Input: dimensioned drawing with shaded views. Units: mm. Origin: part minimum x, y, z. A direction names the side the tool comes from. Give positions to 0.01 mm unless a question says otherwise; leave off trailing zeros. Loops run counter-clockwise (first coordinate to the right, second up) from the corner with the lowest first, then second, coordinate; pieces in that order, holes last.
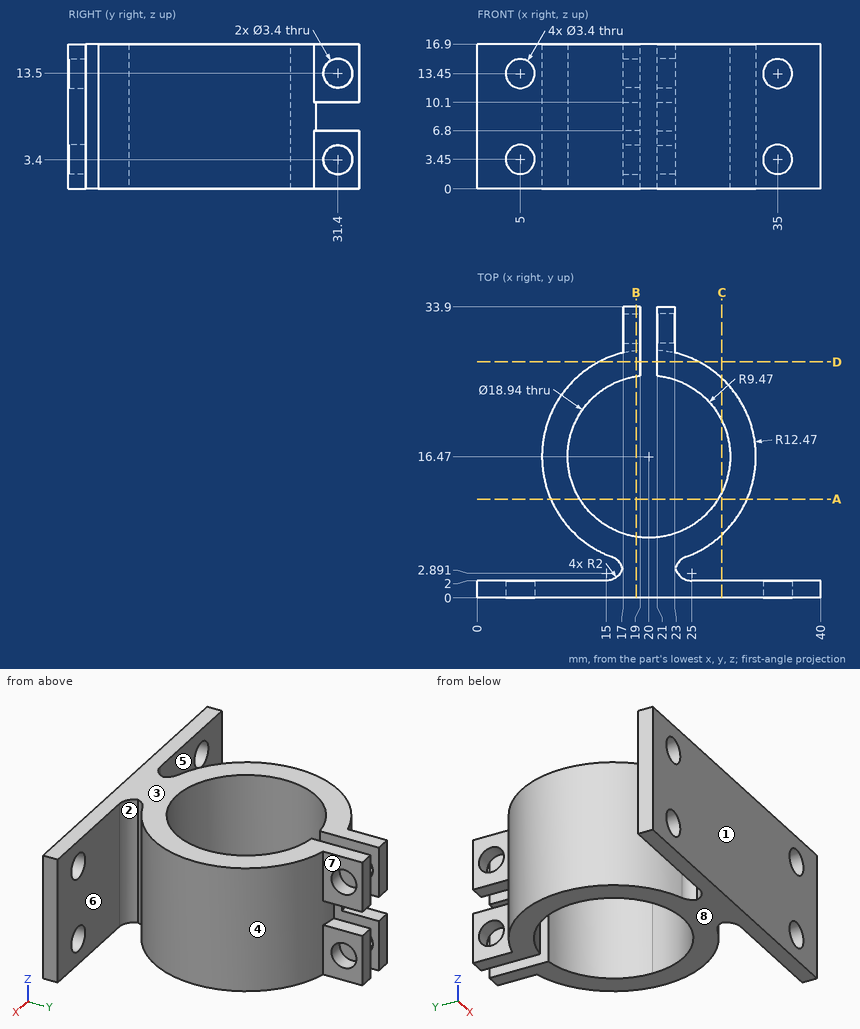
Item 1: Set-up query: the marked faces 5, 6, 7 and 8. Return all of +Z, -Z, +X, -X, +Y, -Y with unobstructed straight access to the full face (end or side cutting, diameter ignored); none if empty.
Values follow:
face 5: +Z, -Z, -X
face 6: +Z, -Z, +X
face 7: +Z, -Z, +X, +Y
face 8: -Z, +X, -X, +Y, -Y
Item 2: Section query A-A on y = 11.5. Return loops of the section in (x, z).
Values follow:
outline: (8.56, 0) - (11.94, 0) - (11.94, 16.9) - (8.56, 16.9) - close; (28.06, 0) - (31.44, 0) - (31.44, 16.9) - (28.06, 16.9) - close
Item 3: Draft query along Y for the marked faces 1, 2, 3 and 4. Return one class per face: +Y half, -Y half, draft (parallel to the pull), parting line (faces both ways), or undercut.
Values follow:
face 1: -Y half
face 2: undercut
face 3: draft
face 4: undercut
Item 4: Section query D-D on y = 27.5. Return loops of the section in (x, z).
Values follow:
outline: (14.18, 0) - (19, 0) - (19, 16.9) - (14.18, 16.9) - close; (21, 0) - (25.82, 0) - (25.82, 16.9) - (21, 16.9) - close
Item 5: Ray query, probe 1 along X at (y, z) = (0.7, 13.45); probe 2 along Y at (x, z) = (21.5, 13.5); probe 3 along Y at (x, z) = (13.5, 3.25). Return the intervals inside material, ascending.
Values follow:
probe 1: x = 0 to 3.3, 6.7 to 33.3, 36.7 to 40
probe 2: y = 0 to 7.12, 25.82 to 29.7, 33.1 to 33.9
probe 3: y = 0 to 2, 5.83 to 9.58, 23.36 to 27.11
Item 6: Section query B-B on x = 18.5. Return loops of the section in (y, z), plus the area to 3 significant figures.
Values follow:
outline: (0, 0) - (7.12, 0) - (7.12, 16.9) - (0, 16.9) - close; (25.82, 0) - (33.9, 0) - (33.9, 6.8) - (28.85, 6.8) - (28.85, 10.1) - (33.9, 10.1) - (33.9, 16.9) - (25.82, 16.9) - close; hole circle Ø3.4 at (31.4, 3.4); hole circle Ø3.4 at (31.4, 13.5)
area: 222 mm2
Item 7: Pin query (flat end, axial travel): pin 1 (6.5 mm diameter, centred on y = 30, z = 5, fed in from -X); pin 2 (5.5 mm diameter, centred on y = 31.4, z = 3.4, fed in from +X); pin 3 (2.5 mm diameter, centred on y = 31.4, z = 13.5, fed in from +X); pin 4 (2.5 mm diameter, centred on y = 28, z = 6.5, fed in from +X). Return the tip coordinate at first contact, or that it passes through.
Values follow:
pin 1: stops at x = 12.94
pin 2: stops at x = 23
pin 3: passes through
pin 4: stops at x = 27.06
Item 8: Section query C-C on x = 28.5. Return loops of the section in (y, z) (1 decimal).
Values follow:
outline: (0, 0) - (2, 0) - (2, 16.9) - (0, 16.9) - close; (7.3, 0) - (12.3, 0) - (12.3, 16.9) - (7.3, 16.9) - close; (20.6, 0) - (25.6, 0) - (25.6, 16.9) - (20.6, 16.9) - close
